For this review, use the dimensioned drawing (mm, ordinates from the lowest corner) and the shaded views. A direction names the side the tool comes from. Coordinates: 2 decimals unless noted, no trailing zeros. Loops run counter-clockwise (first coordinate to the right, second up) from the corner with the lowest first, then second, coordinate; pieces in that order, holes last. Notation, with made-up numbers: (50.5, -35) - (63.5, -35) arc R6 ccw to (63.5, -26) - close; hole circle Ø8 at (46.5, 22). An arc over 180 degrees is marked (long way). Use a Markdown table: item, result. Add a question column.
1) Add section A-A, the plane x = 15. Give the boundary of the cut face in (y, z), and give its area (3 significant figures).
2) Add section B-B, the plane z = 25. Give the boundary of the cut face in (x, y), and give its area (3 significant figures).
3) For the marked faces 1 and 2, list the 3-axis set-ups (+Z, -Z, +X, -X, +Y, -Y) from which the entire face can be reached by the end or side of a thin tool; tool diameter is ignored.
4) To check wall thickness, follow L1, parallel to Y at x = 24.5, z = 14; L2, parallel to Z at x = 23.75, y = 2; L3, parallel to Z at x = 3.75, y = 12.5. State the ranges of each line that lie inside material, in increasing order. Write a range as [from, to].
5) Add section C-C, the plane y = 2. Give the boundary of the cut face in (x, z), and give its area (3 significant figures).
6) Clearance check with flat-ended pins moving along their axes: pin 1 (12 mm diameter, centred on x = 15.5, z = 42.5, fed in from -Y); pin 2 (4 mm diameter, centred on y = 2.5, z = 23, fed in from +X). State where each tip first meets the part, or that it passes through.
7) Add section D-D, the plane z = 11.5. Give the boundary of the cut face in (x, y), and give its area (3 significant figures).
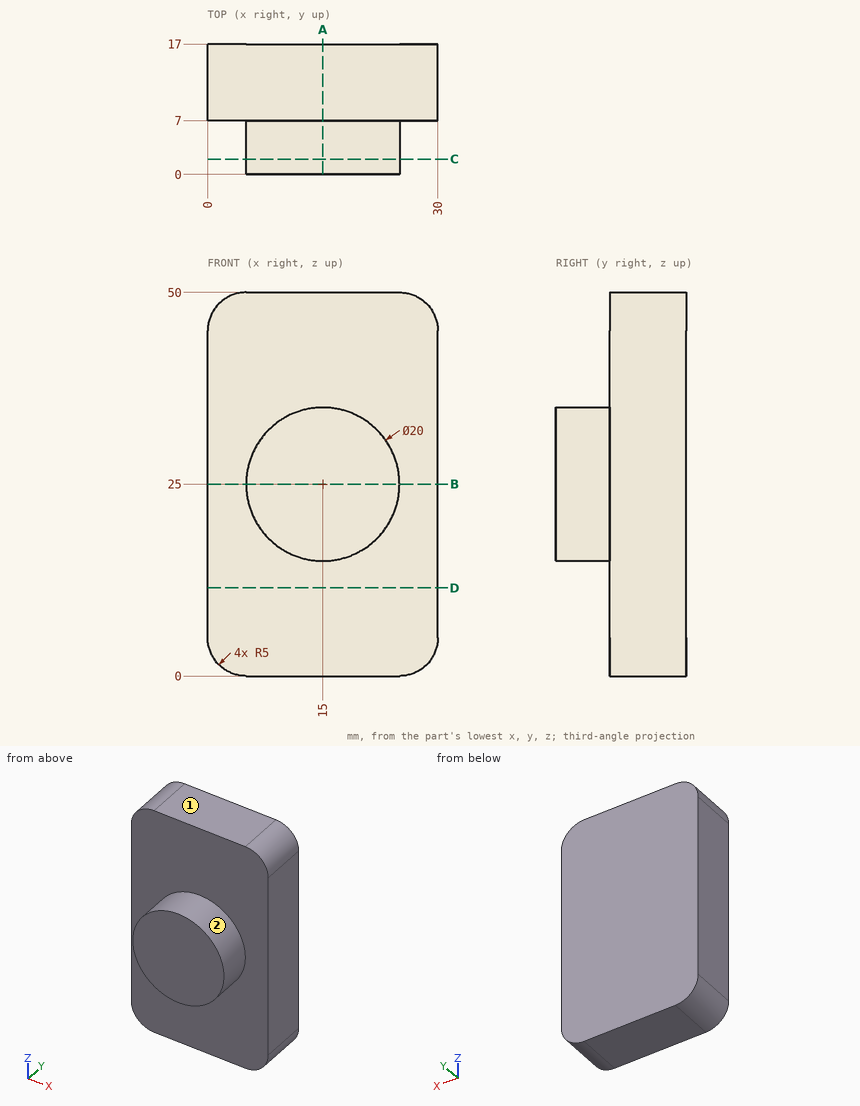
From the geometry:
| question | item | result |
|---|---|---|
| 1 | outline | (0, 15) - (7, 15) - (7, 0) - (17, 0) - (17, 50) - (7, 50) - (7, 35) - (0, 35) - close |
| 1 | area | 640 mm^2 |
| 2 | outline | (0, 7) - (5, 7) - (5, 0) - (25, 0) - (25, 7) - (30, 7) - (30, 17) - (0, 17) - close |
| 2 | area | 440 mm^2 |
| 3 | face 1 | +Z, +X, -X, +Y, -Y |
| 3 | face 2 | -Y |
| 4 | L1 | y = [7, 17] |
| 4 | L2 | z = [20.16, 29.84] |
| 4 | L3 | z = [0.16, 49.84] |
| 5 | outline | circle Ø20 at (15, 25) |
| 5 | area | 314 mm^2 |
| 6 | pin 1 | stops at y = 7 |
| 6 | pin 2 | stops at x = 25 |
| 7 | outline | (0, 7) - (30, 7) - (30, 17) - (0, 17) - close |
| 7 | area | 300 mm^2 |
